Source: CAD feature listing. Evaluate the final solid. Frame: model axes, mm. A direction names the side the tool comes from. Round coordinates to 2 decimals unless told otherwise and drop trailing zeros. Loops run counter-clockwise (first coordinate to the right, second up) from the corner with the lowest first, then second, coordinate; pieces in that order, holes last. Notation, with made-up numbers: M 5,71.25 L 27,71.25 A13 cw 27,77.25 Z; hole C 66,25 d3. An arc over 180 degrees is marked long. One line per item, written item: value.
from build123d import *

# Parameters (mm, degrees)
F0_W     = 152.4
F0_H     = 1066.8
F0_W_2   = 114.3
F0_H_2   = 1028.7
F1_DEPTH = 704.85
F3_DEPTH = 25.4
F5_DEPTH = 25.4


# Not quite as in the source:
# - a feature names something its author has since deleted; it is built from what else it names


with BuildPart() as f1:
    # F0 (on Top) → F1 (new body)
    with BuildSketch(Plane.XY):
        Rectangle(F0_W, F0_H)
        Rectangle(F0_W_2, F0_H_2, mode=Mode.SUBTRACT)
    extrude(amount=F1_DEPTH)

    # F2 (on face) → F3 (cut)
    with BuildSketch(Plane.YZ.offset(76.2)):
        with BuildLine():
            ThreePointArc((30.226, 596.9), (-21.3730095681, 618.2730095681), (0, 566.674))
            ThreePointArc((0, 566.674), (21.3730095681, 575.5269904319), (30.226, 596.9))
        make_face()
        Polygon((-133.35, 101.6), (0, 101.6), (133.35, 101.6), (133.35, 419.1), (0, 419.1), (-133.35, 419.1), align=None)
    extrude(amount=-F3_DEPTH, mode=Mode.SUBTRACT)

    # F4 (on face) → F5 (cut)
    with BuildSketch(Plane(origin=(-76.2, 0, 0), x_dir=(0, -1, 0), z_dir=(-1, 0, 0))):
        with BuildLine():
            ThreePointArc((30.226, 406.4), (-21.3730095681, 427.7730095681), (0, 376.174))
            ThreePointArc((0, 376.174), (21.3730095681, 385.0269904319), (30.226, 406.4))
        make_face()
    extrude(amount=-F5_DEPTH, mode=Mode.SUBTRACT)


solid = f1.part
1. Section query C-C (y = 102). Return the cut outline in (x, z), and give its area (3 significant figures).
Report:
outline: M -76.2,0 L -57.15,0 L -57.15,704.85 L -76.2,704.85 Z; M 57.15,0 L 76.2,0 L 76.2,101.6 L 57.15,101.6 Z; M 57.15,419.1 L 76.2,419.1 L 76.2,704.85 L 57.15,704.85 Z
area: 20,800 mm2
2. Reachability of faces 1 (the face through (-62, 82, 0)), 2 (the face through (-57.15, -7, 347)) from +Z, -Z, +X, -X, +Y, -Y: full face, straight path, thin tool, end or side. Return the list, or none.
Report:
face 1: -Z, +X, -X, +Y, -Y
face 2: +Z, -Z
3. Section query B-B (x = -13). Return the cut outline in (y, z).
Report:
outline: M -533.4,0 L -514.35,0 L -514.35,704.85 L -533.4,704.85 Z; M 514.35,0 L 533.4,0 L 533.4,704.85 L 514.35,704.85 Z
4. Ray query, line 1 (Z direction, x = 62.75, y = 0); line 2 (Y direction, x = -64, z = 406); line 3 (X direction, y = -339, z = 483). Return the intervals inside material, ascending. Write a range as [from, to].
Report:
line 1: z = [0, 101.6], [419.1, 566.67], [627.13, 704.85]
line 2: y = [-533.4, -30.22], [30.22, 533.4]
line 3: x = [-76.2, -57.15], [57.15, 76.2]
5. Pull-direction query (X, two-part tool) for faces 3 (the face through (57.15, -7, 426)), 4 (the face through (-76.2, -7, 347)), 5 (the face through (-1, -533.4, 347)), 6 (the face through (76.2, -7, 426)); classes: released by +X, released by -X, zero draft, split by the parting line, or undercut.
Report:
face 3: undercut
face 4: released by -X
face 5: zero draft
face 6: released by +X
6. Section query A-A (y = 393.5). Return the cut outline in (x, z).
Report:
outline: M -76.2,0 L -57.15,0 L -57.15,704.85 L -76.2,704.85 Z; M 57.15,0 L 76.2,0 L 76.2,704.85 L 57.15,704.85 Z
7. Section query D-D (z = 493). Return the cut outline in (x, y).
Report:
outline: M -76.2,-533.4 L 76.2,-533.4 L 76.2,533.4 L -76.2,533.4 Z; hole M -57.15,-514.35 L 57.15,-514.35 L 57.15,514.35 L -57.15,514.35 Z
